The drawing under review shows one solid part. Ordinate dimensions are in mm from its lowest x, y, z. A direction names the side the tool comes from. Give positions to 0.01 mm unless a question says otherwise; leave off trailing zeros. Write each loop counter-clockwise with the first axis right and the second up, starting at its lowest first coordinate (ties: lowest second). Pieces come first, ordered by that corner, then holes.
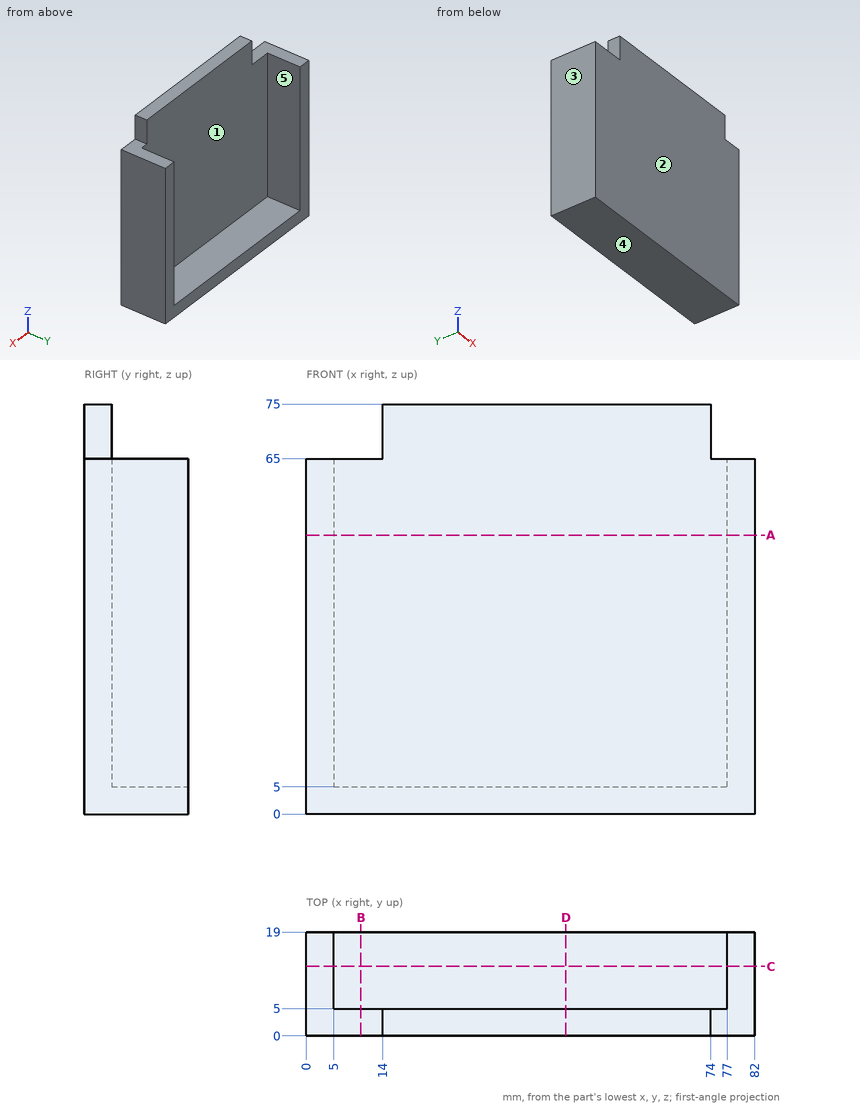
1) To check wall thickness, follow probe 1 along X at (y, z) = (6, 34.5); probe 2 along Z at (x, y) = (54, 13.25). State the ranges of each line that lie inside material, in increasing order.
2) The part is to be moulded in two halves that separate along X. For the marked faces 3, 4 and 5, say which applies: +X half, -X half, draft (parallel to the pull), parting line (faces both ways), or undercut.
3) Consider section A-A, the plane z = 51. Give the boundary of the cut face in (x, y), then the cut area to 3 significant figures.
4) Consider section D-D, the plane x = 47.5. Give the boundary of the cut face in (y, z), then the cut area to 3 significant figures.
5) Insertion check: pin 1 (4 mm diameter, centred on x = 26, z = 23.5, fed in from +Y); pin 2 (5.5 mm diameter, centred on y = 2, z = 68.5, fed in from +X); pin 3 (2.5 mm diameter, centred on y = 3.5, z = 72, fed in from -X). Each pin has a flat end and moves straight along its axis. Give the tip position at first contact, or say it passes through.
6) Tool access review of the marked faces 1 and 2: name each direction out of +Z, -Z, +X, -X, +Y, -Y from which nothing blocks a thin tool from reaching the whole face with its end or side.
7) Consider section B-B, the plane x = 10. Give the boundary of the cut face in (y, z), then the cut area to 3 significant figures.
8) Consider section C-C, the plane y = 12.75. Give the boundary of the cut face in (x, z), then the cut area to 3 significant figures.
Answer block:
1. probe 1: x = 0 to 5, 77 to 82
1. probe 2: z = 0 to 5
2. face 3: -X half
2. face 4: draft
2. face 5: undercut
3. outline: (0, 0) - (82, 0) - (82, 19) - (77, 19) - (77, 5) - (5, 5) - (5, 19) - (0, 19) - close
3. area: 550 mm2
4. outline: (0, 0) - (19, 0) - (19, 5) - (5, 5) - (5, 75) - (0, 75) - close
4. area: 445 mm2
5. pin 1: stops at y = 5
5. pin 2: stops at x = 74
5. pin 3: stops at x = 14
6. face 1: +Z, +Y
6. face 2: +Z, -Z, +X, -X, -Y
7. outline: (0, 0) - (19, 0) - (19, 5) - (5, 5) - (5, 65) - (0, 65) - close
7. area: 395 mm2
8. outline: (0, 0) - (82, 0) - (82, 65) - (77, 65) - (77, 5) - (5, 5) - (5, 65) - (0, 65) - close
8. area: 1,010 mm2
